```python
from build123d import *

# Parameters (mm, degrees)
F1_DEPTH       = 16
F2_W           = 10
F2_H           = 11.5
F3_DEPTH       = 30.001
F4_W           = 10
F4_H           = 4
F5_DEPTH       = 16.001
F7_D           = 2.5
F7_DEPTH       = 10
F7_TIP         = 0.7510757738
F9_D           = 4.5
F9_DEPTH       = 10
F9_CBORE_D     = 8
F9_CBORE_DEPTH = 4.4
F9_TIP         = 1.3519363928
F10_R          = 5
F11_DEPTH      = 1


with BuildPart() as f1:
    # F0 (on Front) → F1 (new body)
    with BuildSketch(Plane.XZ):
        Polygon((14, 30), (0, 30), (-14, 30), (-14, 10), (-30, 10), (-30, 0), (0, 0), (30, 0), (30, 10), (14, 10), align=None)
    extrude(amount=F1_DEPTH)

    # F2 (on face) → F3 (cut, through all)
    with BuildSketch(Plane.XY.offset(30)):
        with Locations((0, -10.25)):
            Rectangle(F2_W, F2_H)
    extrude(amount=-F3_DEPTH, mode=Mode.SUBTRACT)

    # F4 (on face) → F5 (cut, through all)
    with BuildSketch(Plane(origin=(0, 0, 0), x_dir=(-1, 0, 0), z_dir=(0, 1, 0))):
        with Locations((0, 2)):
            Rectangle(F4_W, F4_H)
    extrude(amount=-F5_DEPTH, mode=Mode.SUBTRACT)

    # F7
    with Locations(Plane.XZ.offset(16)):
        with Locations((10, 26), (-10, 10)):
            Hole(F7_D / 2, depth=F7_DEPTH)
            with Locations((0, 0, -(F7_DEPTH + F7_TIP / 2))):  # 118° drill point
                Cone(0, F7_D / 2, F7_TIP, mode=Mode.SUBTRACT)

    # F9
    with Locations(Plane.XY.offset(10)):
        with Locations((22.5, -8), (-22.5, -8)):
            CounterBoreHole(F9_D / 2, F9_CBORE_D / 2, F9_CBORE_DEPTH, depth=F9_DEPTH)
            with Locations((0, 0, -(F9_DEPTH + F9_TIP / 2))):  # 118° drill point
                Cone(0, F9_D / 2, F9_TIP, mode=Mode.SUBTRACT)

    # F10 (on face) → F11 (cut)
    with BuildSketch(Plane(origin=(0, 0, 0), x_dir=(-1, 0, 0), z_dir=(0, 1, 0))):
        with Locations((0, 11)):
            Circle(F10_R)
    extrude(amount=-F11_DEPTH, mode=Mode.SUBTRACT)


solid = f1.part
```
Verification items for the finished model (mm, model axes). A direction names the side the tool comes from. Coordinates: 2 decimals unless noted, no trailing zeros. Write each loop counter-clockwise with the first axis right and the second up, starting at its lowest first coordinate (ties: lowest second). Pieces come first, ordered by that corner, then holes. Notation, with made-up numbers: M 59,0.5 L 99,0.5 A26 cw 99,30.5 Z; hole C 77,13 d8. An arc over 180 degrees is marked long. One line per item, written item: value.
Item 1: Section check C-C, the plane x = 0. Record the boundary of the cut face in (y, z), plus the area to 3 significant figures.
Check sheet entries:
outline: M -4.5,4 L 0,4 L 0,6 L -1,6 L -1,16 L 0,16 L 0,30 L -4.5,30 Z
area: 107 mm^2
Item 2: Mould release check, pull along Z, two halves, no side actions. Record for faces 4 (the cylindrical face through (19.3, -10.4, 7.8)), 5 (the cylindrical face through (-9.079, -10.93, 10.845)), 6 (the flat face through (0, -2, 4)): pulls with the +Z half, pulls with the -Z half, needs draft (parallel to the pull), parting line crosses it, or undercut.
Check sheet entries:
face 4: needs draft
face 5: undercut
face 6: pulls with the -Z half
Item 3: Section check A-A, the plane x = -22.5. Record the boundary of the cut face in (y, z).
Check sheet entries:
outline: M -16,0 L -10.25,0 L -10.25,5.6 L -12,5.6 L -12,10 L -16,10 Z; M -5.75,0 L 0,0 L 0,10 L -4,10 L -4,5.6 L -5.75,5.6 Z
Item 4: Access from +Z, -Z, +X, -X, +Y, -Y to the whole of each face (thin tool, end or side, straight path). Record for faces 1 (the flat face through (-18, -8, 10)), 2 (the flat face through (-21, -10, 5.6)), 3 (the cylindrical face through (0.651, -0.493, 15.957)).
Check sheet entries:
face 1: +Z, -X, +Y, -Y
face 2: +Z
face 3: +Y
Item 5: Section check B-B, the plane y = -7.25. State how many separate pieces and enclosed holes the cut face has, plus the area to 3 significant figures.
Check sheet entries:
separate pieces: 4
enclosed holes: 2
area: 734 mm^2
Item 6: Gauge pin test, flat ends, axial feed: pin 1 Ø6.5 at (x, y) = (22.5, -8) entering from +Z; pin 2 Ø8 at (x, y) = (25, -8) entering from +Z; pin 3 Ø3.5 at (x, y) = (-2.5, -2) entering from -Z. Record the tip position at first contact, or that the pin passes through.
Check sheet entries:
pin 1: stops at z = 5.6
pin 2: stops at z = 10
pin 3: stops at z = 4
Item 7: Section check D-D, the plane z = 19.5. Record the boundary of the cut face in (x, y).
Check sheet entries:
outline: M -14,-16 L -5,-16 L -5,-4.5 L 5,-4.5 L 5,-16 L 14,-16 L 14,0 L -14,0 Z
Item 8: Scan lines: line 1 along Y through (x, z) = (22.5, 3.6); line 2 along X through (y, z) = (-9, 22.25); line 3 along Z through (x, y) = (10, -13.25). Record each from-to range of solid material in increasing order.
Check sheet entries:
line 1: y = -16 to -10.25, -5.75 to 0
line 2: x = -14 to -5, 5 to 14
line 3: z = 0 to 24.75, 27.25 to 30
